For this review, take the finished solid that the model builds, in its own axes (mm). A direction names the side the tool comes from. Give positions to 0.01 mm unless a question says otherwise; leave off trailing zeros. Write each loop counter-clockwise with the first axis right and the second up, starting at its lowest first coordinate (ties: lowest second). Pieces come first, ordered by that corner, then holes. Notation, with made-up numbers: M -17.5,-27 L 37.5,-27 A35 cw 37.5,11 Z; hole C 77,14.25 d3. An arc over 180 degrees is marked long. Use one line per item in the form item = value. Start each with the question number.
Q1. Consider section D-D on z = -74. Write out the cut boundary in (x, y).
Q2. Clearance check with flat-ended pins moving along their axes: pin 1 Ø5 at (x, z) = (96, -14.5) entering from -Y; pin 2 Ø19 at (x, z) = (25.5, -60) entering from +Y; pin 3 Ø15 at (x, z) = (71, -75.5) entering from +Y; pin 4 Ø2 at (y, z) = (85.5, -37) entering from +X. State where each tip first meets the part, or that it passes through.
Q3. Consider section A-A on x = 127. Write out the cut boundary in (y, z) (3 decimals), and give its area (3 significant figures).
Q4. Mouldability with a two-part tool opening along X and no side actions: class faces 1 (the flat face through (165.28, 56.35, -85.32)), 2 (the flat face through (101.6, 99, -56)), 3 (the flat face through (0, 56, -58)), 4 (the flat face through (77, 56, -114.3)) as released by +X, released by -X, zero draft, split by the parting line, or undercut.
Q5. Tool access review of faces 5 (the flat face through (50.8, 99, -56)), 6 (the flat face through (140, 101.6, -57)), 7 (the flat face through (25, 114.3, -19)): name each direction out of +Z, -Z, +X, -X, +Y, -Y from which nothing blocks a thin tool from reaching the whole face with its end or side.
Q6. Consider section B-B on y = 96. Write out the cut boundary in (x, z) (3 decimals), and give its area (3 significant figures).
Q7. For probe 1 along X at (y, z) = (81, -57.15) (3 decimals); probe 2 along Z at (x, y) = (127, 23) (3 decimals); probe 3 along X at (y, z) = (75, -57), list the stretches that pass through material, from the lowest coordinate up. Write a range as [from, to].
Q8. Consider section C-C on y = 7.5. Write out the cut boundary in (x, z) (3 decimals).
```python
from build123d import *

# Parameters (mm, degrees)
BOSS_EXTRUDE1_DEPTH = 114.3
CUT_EXTRUDE4_DEPTH  = 12.7
SKETCH5_W           = 50.8
SKETCH5_H           = 114.3
CUT_EXTRUDE5_DEPTH  = 25.4
SKETCH6_R           = 9.525
CUT_EXTRUDE6_DEPTH  = 2286
SKETCH7_R           = 9.525
CUT_EXTRUDE7_DEPTH  = 2286


with BuildPart() as part:
    # Sketch2 → Boss-Extrude1 (new body)
    with BuildSketch(Plane(origin=(0, 0, 0), x_dir=(1, 0, 0), z_dir=(0, 1, 0))):
        Polygon((0, 0), (152.4, 0), (177.8, 57.15), (152.4, 114.3), (0, 114.3), align=None)
    extrude(amount=BOSS_EXTRUDE1_DEPTH)

    # Sketch3 → Cut-Extrude4 (cut)
    with BuildSketch(Plane(origin=(0, 114.3, 0), x_dir=(1, 0, 0), z_dir=(0, 1, 0))):
        Polygon((169.333333333, 38.1), (0, 38.1), (0, 76.2), (267.804009423, 76.2), (218.011692499, 38.1), align=None)
    extrude(amount=-CUT_EXTRUDE4_DEPTH, mode=Mode.SUBTRACT)

    # Sketch5 → Cut-Extrude5 (cut)
    with BuildSketch(Plane(origin=(0, 114.3, 0), x_dir=(1, 0, 0), z_dir=(0, 1, 0))):
        with Locations((76.2, 57.15)):
            Rectangle(SKETCH5_W, SKETCH5_H)
    extrude(amount=-CUT_EXTRUDE5_DEPTH, mode=Mode.SUBTRACT)

    # Sketch6 → Cut-Extrude6 (cut)
    with BuildSketch(Plane(origin=(0, 101.6, 0), x_dir=(1, 0, 0), z_dir=(0, 1, 0))):
        with Locations((127, 57.15)):
            Circle(SKETCH6_R)
    extrude(amount=-CUT_EXTRUDE6_DEPTH, mode=Mode.SUBTRACT)

    # Sketch7 → Cut-Extrude7 (cut)
    with BuildSketch(Plane(origin=(0, 101.6, 0), x_dir=(1, 0, 0), z_dir=(0, 1, 0))):
        with Locations((25.4, 57.15)):
            Circle(SKETCH7_R)
    extrude(amount=-CUT_EXTRUDE7_DEPTH, mode=Mode.SUBTRACT)


solid = part.part
```
Working result:
q1.outline = M 0,0 L 170.31,0 L 170.31,101.6 L 101.6,101.6 L 101.6,88.9 L 50.8,88.9 L 50.8,101.6 L 0,101.6 Z
q2.pin_1 = 0
q2.pin_2 = 101.6
q2.pin_3 = 88.9
q2.pin_4 = 169.29
q3.outline = M 0,-114.3 L 114.3,-114.3 L 114.3,-76.2 L 101.6,-76.2 L 101.6,-66.675 L 0,-66.675 Z; M 0,-47.625 L 101.6,-47.625 L 101.6,-38.1 L 114.3,-38.1 L 114.3,0 L 0,0 Z
q3.area = 10,600 mm²
q4.face_1 = released by +X
q4.face_2 = undercut
q4.face_3 = released by -X
q4.face_4 = zero draft
q5.face_5 = +Z, -Z, +Y
q5.face_6 = +X, -X, +Y
q5.face_7 = +Z, -Z, +X, -X, +Y
q6.outline = M 0,-114.3 L 50.8,-114.3 L 50.8,0 L 0,0 Z; M 101.6,-114.3 L 152.4,-114.3 L 177.8,-57.15 L 152.4,0 L 101.6,0 Z; hole C 25.4,-57.15 d19.05; hole C 127,-57.15 d19.05
q6.area = 12,500 mm²
q7.probe_1 = [0, 15.875], [34.925, 117.475], [136.525, 177.8]
q7.probe_2 = [-114.3, -66.675], [-47.625, 0]
q7.probe_3 = [0, 15.88], [34.92, 117.48], [136.52, 177.73]
q8.outline = M 0,-114.3 L 152.4,-114.3 L 177.8,-57.15 L 152.4,0 L 0,0 Z; hole C 25.4,-57.15 d19.05; hole C 127,-57.15 d19.05
